from build123d import *

# Parameters (mm, degrees)
SKETCH_1_R      = 3.1
SKETCH_1_W      = 167
SKETCH_1_H      = 146
EXTRUDE_1_DEPTH = 2


with BuildPart() as part:
    # 草图1 → 凸台-拉伸1 (new body)
    # profile 1 of 4: a face of its own
    with BuildSketch(Plane(origin=(0, 0, 0), x_dir=(1, 0, 0), z_dir=(0, 1, 0))):
        Polygon((-154.747658954, 153.385197935), (-154.747658954, 33.385197935), (-214.747658954, 33.385197935), (-214.747658954, -126.614802065), (-14.747658954, -126.614802065), (-14.747658954, -96.614802065), (105.252341046, -96.614802065), (105.252341046, -126.614802065), (305.252341046, -126.614802065), (305.252341046, 33.385197935), (245.252341046, 33.385197935), (245.252341046, 153.385197935), align=None)
        with Locations(Location((-199.747658954, -11.614802065, 0), (0, 0, 270))):
            Circle(SKETCH_1_R, mode=Mode.SUBTRACT)
        with Locations(Location((-169.747658954, -11.614802065, 0), (0, 0, 270))):
            Circle(SKETCH_1_R, mode=Mode.SUBTRACT)
        with Locations(Location((-199.747658954, 18.385197935, 0), (0, 0, 270))):
            Circle(SKETCH_1_R, mode=Mode.SUBTRACT)
        with Locations(Location((-169.747658954, 18.385197935, 0), (0, 0, 270))):
            Circle(SKETCH_1_R, mode=Mode.SUBTRACT)
        with Locations(Location((-139.747658954, 108.385197935, 0), (0, 0, 270))):
            Circle(SKETCH_1_R, mode=Mode.SUBTRACT)
        with Locations(Location((-109.747658954, 108.385197935, 0), (0, 0, 270))):
            Circle(SKETCH_1_R, mode=Mode.SUBTRACT)
        with Locations(Location((-139.747658954, 138.385197935, 0), (0, 0, 270))):
            Circle(SKETCH_1_R, mode=Mode.SUBTRACT)
        with Locations(Location((-109.747658954, 138.385197935, 0), (0, 0, 270))):
            Circle(SKETCH_1_R, mode=Mode.SUBTRACT)
        with Locations(Location((260.252341046, -11.614802065, 0), (0, 0, 270))):
            Circle(SKETCH_1_R, mode=Mode.SUBTRACT)
        with Locations(Location((290.252341046, -11.614802065, 0), (0, 0, 270))):
            Circle(SKETCH_1_R, mode=Mode.SUBTRACT)
        with Locations(Location((260.252341046, 18.385197935, 0), (0, 0, 270))):
            Circle(SKETCH_1_R, mode=Mode.SUBTRACT)
        with Locations(Location((290.252341046, 18.385197935, 0), (0, 0, 270))):
            Circle(SKETCH_1_R, mode=Mode.SUBTRACT)
        with Locations(Location((200.252341046, 108.385197935, 0), (0, 0, 270))):
            Circle(SKETCH_1_R, mode=Mode.SUBTRACT)
        with Locations(Location((230.252341046, 108.385197935, 0), (0, 0, 270))):
            Circle(SKETCH_1_R, mode=Mode.SUBTRACT)
        with Locations(Location((200.252341046, 138.385197935, 0), (0, 0, 270))):
            Circle(SKETCH_1_R, mode=Mode.SUBTRACT)
        with Locations(Location((230.252341046, 138.385197935, 0), (0, 0, 270))):
            Circle(SKETCH_1_R, mode=Mode.SUBTRACT)
    # profile 2 of 4: a face of its own
    with BuildSketch(Plane(origin=(0, 0, 0), x_dir=(1, 0, 0), z_dir=(0, 1, 0))):
        Polygon((-14.747658954, -186.614802065), (-214.747658954, -186.614802065), (-214.747658954, -346.614802065), (-154.747658954, -346.614802065), (-154.747658954, -466.614802065), (245.252341046, -466.614802065), (245.252341046, -346.614802065), (305.252341046, -346.614802065), (305.252341046, -186.614802065), (105.252341046, -186.614802065), (105.252341046, -216.614802065), (-14.747658954, -216.614802065), align=None)
        with Locations(Location((-139.747658954, -451.614802065, 0), (0, 0, 270))):
            Circle(SKETCH_1_R, mode=Mode.SUBTRACT)
        with Locations(Location((-109.747658954, -451.614802065, 0), (0, 0, 270))):
            Circle(SKETCH_1_R, mode=Mode.SUBTRACT)
        with Locations(Location((-139.747658954, -421.614802065, 0), (0, 0, 270))):
            Circle(SKETCH_1_R, mode=Mode.SUBTRACT)
        with Locations(Location((-109.747658954, -421.614802065, 0), (0, 0, 270))):
            Circle(SKETCH_1_R, mode=Mode.SUBTRACT)
        with Locations(Location((-199.747658954, -331.614802065, 0), (0, 0, 270))):
            Circle(SKETCH_1_R, mode=Mode.SUBTRACT)
        with Locations(Location((-169.747658954, -331.614802065, 0), (0, 0, 270))):
            Circle(SKETCH_1_R, mode=Mode.SUBTRACT)
        with Locations(Location((-199.747658954, -301.614802065, 0), (0, 0, 270))):
            Circle(SKETCH_1_R, mode=Mode.SUBTRACT)
        with Locations(Location((-169.747658954, -301.614802065, 0), (0, 0, 270))):
            Circle(SKETCH_1_R, mode=Mode.SUBTRACT)
        with Locations((45.252341046, -313.614802065)):
            Rectangle(SKETCH_1_W, SKETCH_1_H, mode=Mode.SUBTRACT)
        with Locations(Location((200.252341046, -451.614802065, 0), (0, 0, 270))):
            Circle(SKETCH_1_R, mode=Mode.SUBTRACT)
        with Locations(Location((230.252341046, -451.614802065, 0), (0, 0, 270))):
            Circle(SKETCH_1_R, mode=Mode.SUBTRACT)
        with Locations(Location((200.252341046, -421.614802065, 0), (0, 0, 270))):
            Circle(SKETCH_1_R, mode=Mode.SUBTRACT)
        with Locations(Location((230.252341046, -421.614802065, 0), (0, 0, 270))):
            Circle(SKETCH_1_R, mode=Mode.SUBTRACT)
        with Locations(Location((260.252341046, -331.614802065, 0), (0, 0, 270))):
            Circle(SKETCH_1_R, mode=Mode.SUBTRACT)
        with Locations(Location((290.252341046, -331.614802065, 0), (0, 0, 270))):
            Circle(SKETCH_1_R, mode=Mode.SUBTRACT)
        with Locations(Location((260.252341046, -301.614802065, 0), (0, 0, 270))):
            Circle(SKETCH_1_R, mode=Mode.SUBTRACT)
        with Locations(Location((290.252341046, -301.614802065, 0), (0, 0, 270))):
            Circle(SKETCH_1_R, mode=Mode.SUBTRACT)
    # profile 3 of 4: a face of its own
    with BuildSketch(Plane(origin=(0, 0, 0), x_dir=(1, 0, 0), z_dir=(0, 1, 0))):
        Polygon((-14.747658954, -126.614802065), (-214.747658954, -126.614802065), (-214.747658954, -186.614802065), (-14.747658954, -186.614802065), (105.252341046, -186.614802065), (305.252341046, -186.614802065), (305.252341046, -126.614802065), (105.252341046, -126.614802065), align=None)
    # profile 4 of 4: a face of its own
    with BuildSketch(Plane(origin=(0, 0, 0), x_dir=(1, 0, 0), z_dir=(0, 1, 0))):
        with Locations((45.252341046, -313.614802065)):
            Rectangle(SKETCH_1_W, SKETCH_1_H)
        with Locations(Location((123.752341046, -263.614802065, 0), (0, 0, 270))):
            Circle(SKETCH_1_R, mode=Mode.SUBTRACT)
        with Locations(Location((-33.247658954, -363.614802065, 0), (0, 0, 270))):
            Circle(SKETCH_1_R, mode=Mode.SUBTRACT)
        with Locations(Location((-33.247658954, -263.614802065, 0), (0, 0, 270))):
            Circle(SKETCH_1_R, mode=Mode.SUBTRACT)
        with Locations(Location((123.752341046, -363.614802065, 0), (0, 0, 270))):
            Circle(SKETCH_1_R, mode=Mode.SUBTRACT)
    extrude(amount=EXTRUDE_1_DEPTH)


solid = part.part
CAD build for the part. Positions are in the model's coordinates, mm. Coordinates: 2 decimals unless noted, no trailing zeros. Write each loop counter-clockwise with the first axis right and the second up, starting at its lowest first coordinate (ties: lowest second). Pieces come first, ordered by that corner, then holes. Notation, with made-up numbers: M -14,-21.5 L 10,-21.5 A20 cw 10,-5.5 Z; hole C 44,36 d5. An arc over 180 degrees is marked long. Answer as a JSON object with one key per item and string values. Group by question number.
1) Wall check: line 1 (Z direction, x = -10, y = 0.55); line 2 (Z direction, x = 230.5, y = 1.35); line 3 (X direction, y = 0.3, z = 13). Give the ranges that are in metal, low to high. Write a range as from..to.
2) Saw through at B-B (z = -89). Write the cut outline in (x, y).
3) Pin check, flat tip, straight feed: pin 1 Ø0.6 at (y, z) = (0.5, 399.5) entering from -X. Stop position of the tip, or through.
4) Saw through at A-A (x = 51.5). Write the cut outline in (y, z).
5) Saw through at C-C (y = 1.45). Give the number of separate pieces and of enclosed holes in the cut face, plus the area to 3 significant figures.
Values follow:
{
 "1": {"line 1": "z = -153.39..96.61, 126.61..186.61, 216.61..466.61", "line 2": "z = -153.39..-141.48, -135.3..-111.48, -105.3..418.52, 424.7..448.52, 454.7..466.61", "line 3": "x = -214.75..-202.52, -196.97..-172.52, -166.97..257.48, 263.03..287.48, 293.03..305.25"},
 "2": {"outline": "M -154.75,0 L 245.25,0 L 245.25,2 L -154.75,2 Z"},
 "3": {"pin 1": "stops at x = -154.75"},
 "4": {"outline": "M 0,-153.39 L 2,-153.39 L 2,96.61 L 0,96.61 Z; M 0,126.61 L 2,126.61 L 2,186.61 L 0,186.61 Z; M 0,216.61 L 2,216.61 L 2,466.61 L 0,466.61 Z"},
 "5": {"separate pieces": "1", "enclosed holes": "38", "area": "285,000 mm2"}
}
